The model under review builds one solid part; all positions refer to its coordinate system, in mm. Round coordinates to 2 decimals unless told otherwise and drop trailing zeros. Write each loop counter-clockwise with the first axis right and the second up, starting at its lowest first coordinate (ties: lowest second). Pieces come first, ordered by that corner, then holes. Notation, with made-up numbers: (-32.5, -34) -> (-1.5, -34) arc R31 ccw to (-1.5, 5) -> close; hole circle Ø7 at (-13, 58.25). An arc over 180 degrees is marked (long way). Return JSON: item names as keys, results as strings. Group by question number.
1. For line 1 along X through (y, z) = (39, 0); line 2 along X through (y, z) = (34, 2); line 3 along Z through (x, y) = (143, 38.5), list the stretches that pass through material, from the lowest coordinate up. Write a range as from..to.
2. Take a section at A-A, the plane z = -98. Write out the cut boundary in (x, y).
3. Clearance check with flat-ended pins moving along their axes: P1, Ø11, axis at x = -168.5, z = -170.5, coming from the +Y side; P2, Ø12, axis at y = 22.5, z = 73.5, coming from the +X side; P3, Ø2, axis at y = 20.5, z = 118, coming from the -X side. State where each tip first meets the part, or that it passes through.
4. Take a section at D-D, the plane z = -272.5. Write out the cut boundary in (x, y), then the cut area to 3 significant figures.
5. Take a section at C-C, the plane y = 28. Give the number of separate pieces and of enclosed holes in the cut face, then the cut area to 3 significant figures.
6. Take a section at B-B, the plane x = 102. Write out the cut boundary in (y, z).
from build123d import *

# Parameters (mm, degrees)
SKETCH1_W          = 97.5
SKETCH1_H          = 30
SKETCH2_R          = 11
CUT_EXTRUDE1_DEPTH = 10
SKETCH3_R          = 6
CUT_EXTRUDE2_DEPTH = 447.486281987


with BuildPart() as part:
    # Sketch1 → Revolve1 (revolve)
    with BuildSketch(Plane(origin=(0, 0, 0), x_dir=(0, 0, -1), z_dir=(1, 0, 0)), mode=Mode.PRIVATE) as revolve1_sk:
        with Locations((-266.250000002, 29.605962764)):
            Rectangle(SKETCH1_W, SKETCH1_H)
    revolve(revolve1_sk.sketch.rotate(Axis((0, -1000, 0), (0, 1, 0)), 180), axis=Axis((0, -1000, 0), (0, 1, 0)))

    # Sketch2 → Cut-Extrude1 (cut)
    with BuildSketch(Plane(origin=(0, 44.605962764, 0), x_dir=(1, 0, 0), z_dir=(0, 1, 0))):
        with Locations(Location((0, 240, 0), (0, 0, 270))):
            Circle(SKETCH2_R)
        with Locations(Location((169.705627485, 169.705627485, 0), (0, 0, 270))):
            Circle(SKETCH2_R)
        with Locations(Location((240, 0, 0), (0, 0, 270))):
            Circle(SKETCH2_R)
        with Locations(Location((169.705627485, -169.705627485, 0), (0, 0, 270))):
            Circle(SKETCH2_R)
        with Locations(Location((0, -240, 0), (0, 0, 270))):
            Circle(SKETCH2_R)
        with Locations(Location((-169.705627485, -169.705627485, 0), (0, 0, 270))):
            Circle(SKETCH2_R)
        with Locations(Location((-240, 0, 0), (0, 0, 270))):
            Circle(SKETCH2_R)
        with Locations(Location((-169.705627485, 169.705627485, 0), (0, 0, 270))):
            Circle(SKETCH2_R)
    extrude(amount=-CUT_EXTRUDE1_DEPTH, mode=Mode.SUBTRACT)

    # Sketch3 → Cut-Extrude2 (cut, through all)
    with BuildSketch(Plane(origin=(0, 44.605962764, 0), x_dir=(1, 0, 0), z_dir=(0, 1, 0))):
        with Locations(Location((0, 240, 0), (0, 0, 270))):
            Circle(SKETCH3_R)
        with Locations(Location((169.705627485, 169.705627485, 0), (0, 0, 270))):
            Circle(SKETCH3_R)
        with Locations(Location((240, 0, 0), (0, 0, 270))):
            Circle(SKETCH3_R)
        with Locations(Location((169.705627485, -169.705627485, 0), (0, 0, 270))):
            Circle(SKETCH3_R)
        with Locations(Location((0, -240, 0), (0, 0, 270))):
            Circle(SKETCH3_R)
        with Locations(Location((-169.705627485, -169.705627485, 0), (0, 0, 270))):
            Circle(SKETCH3_R)
        with Locations(Location((-240, 0, 0), (0, 0, 270))):
            Circle(SKETCH3_R)
        with Locations(Location((-169.705627485, 169.705627485, 0), (0, 0, 270))):
            Circle(SKETCH3_R)
    extrude(amount=-CUT_EXTRUDE2_DEPTH, mode=Mode.SUBTRACT)


solid = part.part
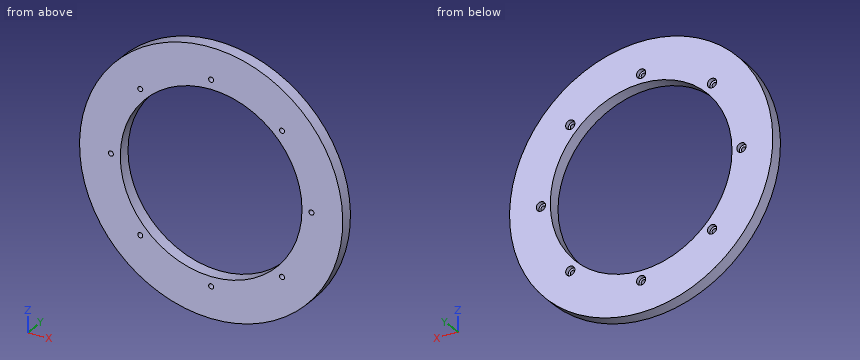
Output:
{
 "1": {"line 1": "x = -315..-251, -229..-217.5, 217.5..229, 251..315", "line 2": "x = -314.99..-245.66, -234.34..-217.49, 217.49..234.34, 245.66..314.99", "line 3": "z = -280.67..-163.88, 163.88..280.67"},
 "2": {"outline": "(-299.37, 14.61) -> (-194.17, 14.61) -> (-194.17, 44.61) -> (-299.37, 44.61) -> close; (194.17, 14.61) -> (299.37, 14.61) -> (299.37, 44.61) -> (194.17, 44.61) -> close"},
 "3": {"P1": "stops at y = 34.61", "P2": "stops at x = 307.68", "P3": "stops at x = -292.47"},
 "4": {"outline": "(-158.02, 14.61) -> (158.02, 14.61) -> (158.02, 44.61) -> (-158.02, 44.61) -> close", "area": "9,480 mm^2"},
 "5": {"separate pieces": "1", "enclosed holes": "9", "area": "162,000 mm^2"},
 "6": {"outline": "(14.61, -298.03) -> (44.61, -298.03) -> (44.61, -192.1) -> (14.61, -192.1) -> close; (14.61, 192.1) -> (44.61, 192.1) -> (44.61, 298.03) -> (14.61, 298.03) -> close"}
}
